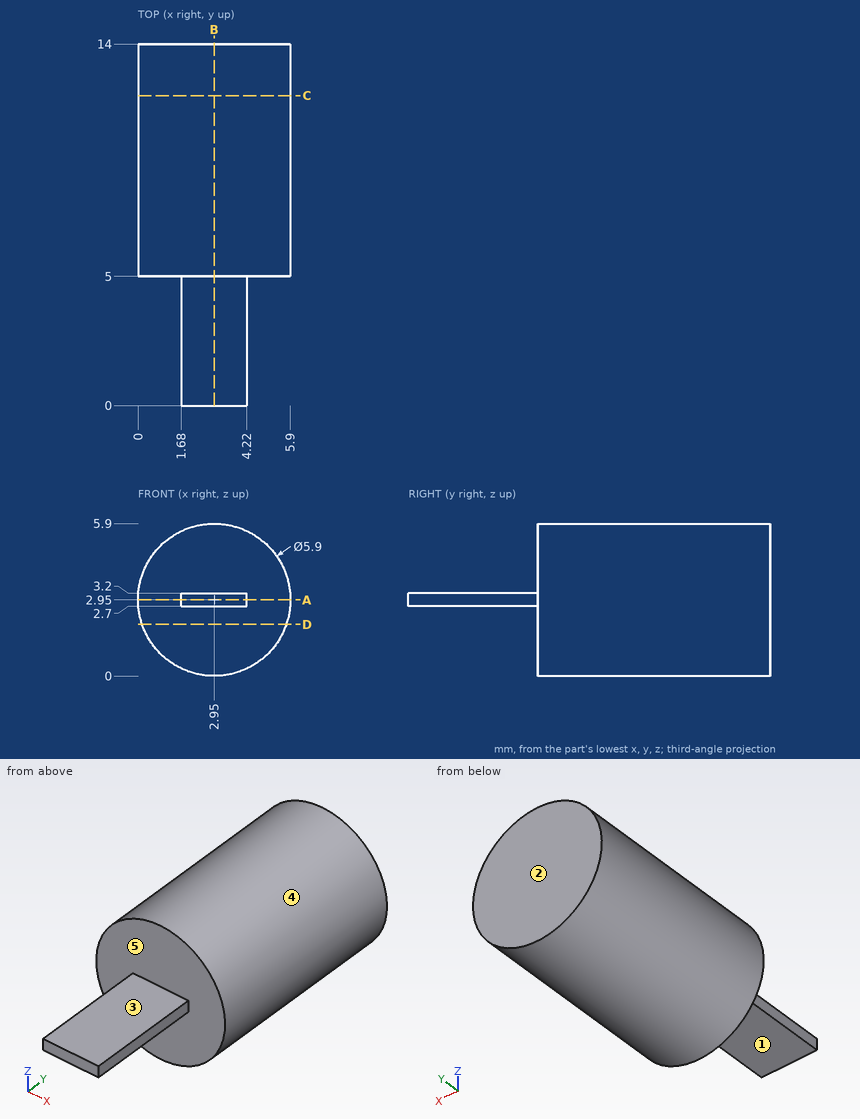
Geometry: see drawing. Coordinates: mm, zero at the bounding-box minimum. A direction names the side the tool comes from. Give positions to 0.01 mm unless a question says otherwise; leave off trailing zeros. Loops run counter-clockwise (first coordinate to the right, second up) from the corner with the lowest first, then second, coordinate; pieces in that order, holes last. Notation, with made-up numbers: (39.5, -28) - (69.5, -28) arc R11 ccw to (69.5, -24) - close; hole circle Ø10 at (1, 67.25). An arc over 180 degrees is marked (long way). Use CSV: the item, a comma, the result in double quotes. Start each with the question number.
Item 1: Mould query, pull axis X, two halves, no side actions, for the marked faces 4 and 5. Classes: pulls with the +X half, pulls with the -X half, needs draft (parallel to the pull), parting line crosses it, or undercut.
Item 2: Reachability of the marked faces 1, 2 and 3 from +Z, -Z, +X, -X, +Y, -Y: full face, straight path, thin tool, end or side. Return the list, or none.
Item 3: Line query: line 1 (Y direction, x = 4.45, z = 3.55); line 2 (Z direction, x = 4.15, y = 3); line 3 (X direction, y = 3, z = 3.1). Output: solid intervals per line, ascending.
Item 4: Contact query for flat-ended pins moving along their axis: P1, Ø2, axis at x = 3.5, y = 2, coming from the +Z side; P2, Ø3, axis at x = 3, y = 2, coming from the -Z side; P3, Ø3, axis at y = 2, z = 2, coming from the +X side. Output: stop coordinate, or through.
Item 5: Section D-D on z = 2. Return loops of the section in (x, y).
Item 6: Section A-A on z = 2.95. Return loops of the section in (x, y).
Item 7: Section C-C on y = 12. Return loops of the section in (x, z), then the cut area to 3 significant figures.
Item 8: Section B-B on x = 2.95. Return loops of the section in (y, z).
Ans:
1,face 4,"parting line crosses it"
1,face 5,"needs draft"
2,face 1,"-Z, +X, -X, -Y"
2,face 2,"+Z, -Z, +X, -X, +Y"
2,face 3,"+Z, +X, -X, -Y"
3,line 1,"y = 5 to 14"
3,line 2,"z = 2.7 to 3.2"
3,line 3,"x = 1.68 to 4.22"
4,P1,"stops at z = 3.2"
4,P2,"stops at z = 2.7"
4,P3,"stops at x = 4.22"
5,outline,"(0.16, 5) - (5.74, 5) - (5.74, 14) - (0.16, 14) - close"
6,outline,"(0, 5) - (1.68, 5) - (1.68, 0) - (4.22, 0) - (4.22, 5) - (5.9, 5) - (5.9, 14) - (0, 14) - close"
7,outline,"circle Ø5.9 at (2.95, 2.95)"
7,area,"27.3 mm2"
8,outline,"(0, 2.7) - (5, 2.7) - (5, 0) - (14, 0) - (14, 5.9) - (5, 5.9) - (5, 3.2) - (0, 3.2) - close"
